The drawing under review shows one solid part. Ordinate dimensions are in mm from its lowest x, y, z. A direction names the side the tool comes from. Give positions to 0.01 mm unless a question says otherwise; leave off trailing zeros. Loops run counter-clockwise (first coordinate to the right, second up) from the corner with the lowest first, then second, coordinate; pieces in that order, holes last. Notation, with made-up numbers: M 66,9.5 L 88,9.5 A6 cw 88,16.5 Z; hole C 85,23 d1. An arc over 180 degrees is marked long. Answer as CSV lines item,"result".
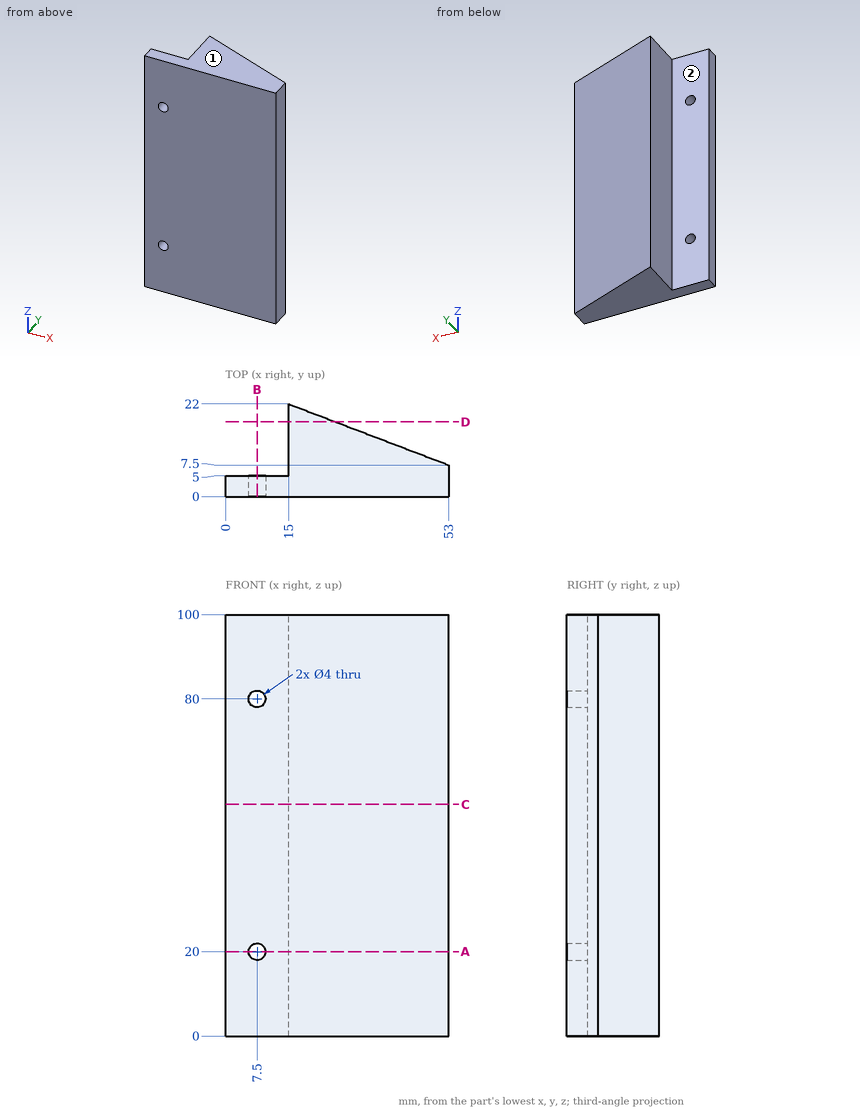
1. We need section A-A, the plane z = 20. Write out the cut boundary in (x, y).
Answer block:
outline,"M 0,0 L 5.5,0 L 5.5,5 L 0,5 Z; M 9.5,0 L 53,0 L 53,7.5 L 15,22 L 15,5 L 9.5,5 Z"
2. For the marked faces 1 and 2, list the 3-axis set-ups (+Z, -Z, +X, -X, +Y, -Y) from which the entire face can be reached by the end or side of a thin tool; tool diameter is ignored.
Answer block:
face 1,"+Z, +X, -X, +Y, -Y"
face 2,"+Z, -Z, -X, +Y"
3. We need section C-C, the plane z = 55. Write out the cut boundary in (x, y), plus the area to 4 significant figures.
Answer block:
outline,"M 0,0 L 53,0 L 53,7.5 L 15,22 L 15,5 L 0,5 Z"
area,"635.5 mm²"
4. For P1, Ø12, axis at x = 7.5, z = 29.5, coming from the +Y side, flat-tipped, find the tip position at first contact; note if it passes through.
Answer block:
P1,"y = 5"
5. To check wall thickness, follow L1, parallel to Z at x = 7.5, y = 2.8; L2, parallel to X at y = 3.8, z = 20; L3, parallel to Y at x = 11, z = 49.5. State the ranges of each line that lie inside material, in increasing order. Write a range as [from, to].
Answer block:
L1,"[0, 18], [22, 78], [82, 100]"
L2,"[0, 5.5], [9.5, 53]"
L3,"[0, 5]"
6. We need section D-D, the plane y = 17.75. Write out the cut boundary in (x, z).
Answer block:
outline,"M 15,0 L 26.14,0 L 26.14,100 L 15,100 Z"
7. We need section B-B, the plane x = 7.5. Write out the cut boundary in (y, z).
Answer block:
outline,"M 0,0 L 5,0 L 5,18 L 0,18 Z; M 0,22 L 5,22 L 5,78 L 0,78 Z; M 0,82 L 5,82 L 5,100 L 0,100 Z"
